from build123d import *

# Parameters (mm, degrees)
EXTRUDE_1_DEPTH             = 4.5
CUT_EXTRUDE_1_DEPTH         = 2.5
SKETCH_2_3_R                = 1.6
CUT_EXTRUDE_2_DEPTH         = 48.8949893
HOLE_WIZARD_M31_D           = 3.2
HOLE_WIZARD_M31_CSINK_D     = 6.2
HOLE_WIZARD_M31_CSINK_ANGLE = 90
SKETCH_7_R                  = 1.6
EXTRUDE_2_DEPTH             = 4.5
EXTRUDE_2_2_DEPTH           = 4.5
FILLET_1_R                  = 1
FILLET_2_R                  = 1
CHAMFER_1_SIZE              = 0.5
CHAMFER_2_SIZE              = 1


with BuildPart() as part:
    # Sketch 1 → Extrude 1 (new body)
    with BuildSketch(Plane.XY):
        with BuildLine():
            Line((42.2, -15), (42.2, 15))
            ThreePointArc((42.2, 15), (40.091168825, 20.091168825), (35, 22.2))
            Line((35, 22.2), (-35, 22.2))
            ThreePointArc((-35, 22.2), (-40.091168825, 20.091168825), (-42.2, 15))
            Line((-42.2, 15), (-42.2, -15))
            ThreePointArc((-42.2, -15), (-40.091168825, -20.091168825), (-35, -22.2))
            Line((-35, -22.2), (35, -22.2))
            ThreePointArc((35, -22.2), (40.091168825, -20.091168825), (42.2, -15))
        make_face()
    extrude(amount=EXTRUDE_1_DEPTH)

    # Sketch 2 → Cut-Extrude 1 (cut)
    with BuildSketch(Plane.XY.offset(4.5)):
        with BuildLine():
            Line((31, -15), (31, -21.2))
            Line((31, -21.2), (-31, -21.2))
            Line((-31, -21.2), (-31, -15))
            ThreePointArc((-31, -15), (-32.171572875, -12.171572875), (-35, -11))
            Line((-35, -11), (-41.2, -11))
            Line((-41.2, -11), (-41.2, 11))
            Line((-41.2, 11), (-35, 11))
            ThreePointArc((-35, 11), (-32.171572875, 12.171572875), (-31, 15))
            Line((-31, 15), (-31, 21.2))
            Line((-31, 21.2), (31, 21.2))
            Line((31, 21.2), (31, 15))
            ThreePointArc((31, 15), (32.171572875, 12.171572875), (35, 11))
            Line((35, 11), (41.2, 11))
            Line((41.2, 11), (41.2, -11))
            Line((41.2, -11), (35, -11))
            ThreePointArc((35, -11), (32.171572875, -12.171572875), (31, -15))
        make_face()
    extrude(amount=-CUT_EXTRUDE_1_DEPTH, mode=Mode.SUBTRACT)

    # Sketch 2_3 → Cut-Extrude 2 (cut, through all)
    with BuildSketch(Plane.XY.offset(4.5)):
        with Locations((-35, -15)):
            Circle(SKETCH_2_3_R)
        with Locations((35, 15)):
            Circle(SKETCH_2_3_R)
        with Locations((35, -15)):
            Circle(SKETCH_2_3_R)
        with Locations((-35, 15)):
            Circle(SKETCH_2_3_R)
    extrude(amount=-CUT_EXTRUDE_2_DEPTH, mode=Mode.SUBTRACT)

    # Hole Wizard M31 (through all)
    with Locations(Plane(origin=(0, 0, 0), x_dir=(-1, 0, 0), z_dir=(0, 0, -1))):
        with Locations((-35, 15), (-35, -15), (35, -15), (35, 15)):
            CounterSinkHole(HOLE_WIZARD_M31_D / 2, HOLE_WIZARD_M31_CSINK_D / 2, counter_sink_angle=HOLE_WIZARD_M31_CSINK_ANGLE)


with BuildPart() as body_2:
    # Sketch 7 → Extrude 2 (new body)
    with BuildSketch(Plane.XY):
        with BuildLine():
            Line((43.473220038, -11.666666667), (50.926779962, -3.333333333))
            ThreePointArc((50.926779962, -3.333333333), (52.2, 0), (50.926779962, 3.333333333))
            Line((50.926779962, 3.333333333), (43.473220038, 11.666666667))
            ThreePointArc((43.473220038, 11.666666667), (42.529138205, 13.215889551), (42.2, 15))
            Line((42.2, 15), (42.2, -15))
            ThreePointArc((42.2, -15), (42.529138205, -13.215889551), (43.473220038, -11.666666667))
        make_face()
        with Locations((47.2, 0)):
            Circle(SKETCH_7_R, mode=Mode.SUBTRACT)
    extrude(amount=EXTRUDE_2_DEPTH)

    # Fillet 1
    fillet_1_edges = [body_2.edges().sort_by_distance(p)[0] for p in [
        (52.2, 0, 4.5),
        (47.2, 7.5, 4.5),
        (42.529138205, 13.215889551, 4.5),
        (42.529138205, -13.215889551, 4.5),
        (47.2, -7.5, 4.5),
    ]]
    fillet(fillet_1_edges, radius=FILLET_1_R)


with BuildPart() as body_3:
    # Sketch 7 → Extrude 2 2 (new body)
    with BuildSketch(Plane.XY):
        with BuildLine():
            Line((-42.2, -15), (-42.2, 15))
            ThreePointArc((-42.2, 15), (-42.529138205, 13.215889551), (-43.473220038, 11.666666667))
            Line((-43.473220038, 11.666666667), (-50.926779962, 3.333333333))
            ThreePointArc((-50.926779962, 3.333333333), (-52.2, 0), (-50.926779962, -3.333333333))
            Line((-50.926779962, -3.333333333), (-43.473220038, -11.666666667))
            ThreePointArc((-43.473220038, -11.666666667), (-42.529138205, -13.215889551), (-42.2, -15))
        make_face()
        with Locations(Location((-47.2, 0, 0), (0, 0, 180))):
            Circle(SKETCH_7_R, mode=Mode.SUBTRACT)
    extrude(amount=EXTRUDE_2_2_DEPTH)

    # Fillet 2
    fillet_2_edges = [body_3.edges().sort_by_distance(p)[0] for p in [
        (-42.529138205, -13.215889551, 4.5),
        (-42.529138205, 13.215889551, 4.5),
        (-47.2, 7.5, 4.5),
        (-52.2, 0, 4.5),
        (-47.2, -7.5, 4.5),
    ]]
    fillet(fillet_2_edges, radius=FILLET_2_R)


with BuildPart() as part_1:
    add(part.part)

    # Combine 1: union body 3, body 2
    add(body_3.part)
    add(body_2.part)

    # Chamfer 1
    chamfer_1_edges = [part_1.edges().sort_by_distance(p)[0] for p in [
        (40.091168825, -20.091168825, 0),
        (-45.6, 0, 0),
        (-52.2, 0, 0),
        (-47.2, -7.5, 0),
        (-42.529138205, -13.215889551, 0),
        (-42.529138205, 13.215889551, 0),
        (-47.2, 7.5, 0),
        (-45.6, 0, 4.5),
        (45.6, 0, 0),
        (42.529138205, -13.215889551, 0),
        (47.2, -7.5, 0),
        (52.2, 0, 0),
        (47.2, 7.5, 0),
        (42.529138205, 13.215889551, 0),
        (45.6, 0, 4.5),
        (-36.6, 15, 4.5),
        (33.4, -15, 4.5),
        (33.4, 15, 4.5),
        (0, -22.2, 0),
        (-36.6, -15, 4.5),
        (-40.091168825, -20.091168825, 0),
        (-40.091168825, 20.091168825, 0),
        (0, 22.2, 0),
        (40.091168825, 20.091168825, 0),
    ]]
    chamfer(chamfer_1_edges, length=CHAMFER_1_SIZE)

    # Chamfer 2
    chamfer_2_edges = [part_1.edges().sort_by_distance(p)[0] for p in [
        (41.2, 11, 3.25),
        (41.2, -11, 3.25),
        (32.171572875, -12.171572875, 2),
        (31, -21.2, 3.25),
        (-31, -21.2, 3.25),
        (-41.2, -11, 3.25),
        (-41.2, 11, 3.25),
        (-31, 21.2, 3.25),
        (31, 21.2, 3.25),
        (32.171572875, 12.171572875, 2),
        (41.2, 0, 2),
        (38.1, -11, 2),
        (31, -18.1, 2),
        (0, -21.2, 2),
        (-31, -18.1, 2),
        (-32.171572875, -12.171572875, 2),
        (-38.1, -11, 2),
        (-41.2, 0, 2),
        (-38.1, 11, 2),
        (-32.171572875, 12.171572875, 2),
        (-31, 18.1, 2),
        (0, 21.2, 2),
        (31, 18.1, 2),
        (38.1, 11, 2),
    ]]
    chamfer(chamfer_2_edges, length=CHAMFER_2_SIZE)


solid = part_1.part
For this review, take the finished solid that the model builds, in its own axes (mm). A direction names the side the tool comes from. Round coordinates to 2 decimals unless told otherwise and drop trailing zeros. Loops run counter-clockwise (first coordinate to the right, second up) from the corner with the lowest first, then second, coordinate; pieces in that order, holes last. Notation, with made-up numbers: (-39, 15.5) - (5, 15.5) arc R18 cw to (5, 33.5) - close; hole circle Ø3 at (-26, -33.5). An arc over 180 degrees is marked (long way). One line per question, with ' | ' between items.
Q1. The part is to be moulded in two halves that separate along X. For faces 1 (the cylindrical face through (40.15, 20.03, 2.47)), 2 (the cylindrical face through (-32.141, -12.203, 3.76)), 3 (the cylindrical face through (-35.208, 16.586, 2.768)), 4 (the cylindrical face through (-42.54, -13.19, 1.98)), say which applies: released by +X, released by -X, zero draft, split by the parting line, or undercut.
Taken from the geometry:
face 1: released by +X | face 2: undercut | face 3: undercut | face 4: released by -X
Q2. Take a section at A-A (x = 0.5). Give the boundary of the cut face in (y, z), and give its area (4 significant figures).
Taken from the geometry:
outline: (-22.2, 0.5) - (-21.7, 0) - (21.7, 0) - (22.2, 0.5) - (22.2, 4.5) - (21.2, 4.5) - (21.2, 3) - (20.2, 2) - (-20.2, 2) - (-21.2, 3) - (-21.2, 4.5) - (-22.2, 4.5) - close | area: 94.55 mm²
Q3. For pin 1 (0.8 mm diameter, centred on y = -2.5, z = 3.5, fed in from +X); pin 2 (0.8 mm diameter, centred on y = -18, z = 4, fed in from +X); pin 3 (10 mm diameter, centred on x = -0.5, y = -6, fed in from +Z), all flat-tipped, find the tip position at first contact; note any pin that passes through.
Taken from the geometry:
pin 1: stops at x = 51.74 | pin 2: stops at x = 41.71 | pin 3: stops at z = 2
Q4. Tool access review of faces 5 (the cylindrical face through (32.141, 12.203, 3.76)), 6 (the flat face through (-47.068, -7.277, 0.253)): name each direction out of +Z, -Z, +X, -X, +Y, -Y from which nothing blocks a thin tool from reaching the whole face with its end or side.
Taken from the geometry:
face 5: +Z | face 6: -Z, -X, -Y
Q5. For line 1 along X through (y, z) = (15, 3.05); line 2 along Y through (x, z) = (-35, 3.3); line 3 along Y through (x, z) = (-35, 2.8), list the stretches that pass through material, from the lowest coordinate up. Write a range as [from, to].
Taken from the geometry:
line 1: x = [-42.2, -36.6], [-33.4, -31], [31, 33.4], [36.6, 42.2] | line 2: y = [-22.2, -16.6], [-13.4, -11], [11, 13.4], [16.6, 22.2] | line 3: y = [-22.2, -16.6], [-13.4, -10.8], [10.8, 13.4], [16.6, 22.2]
